Design review of the part shown in the three views and the two pictorial views. Dimensions are in mm from the part's minimum x, y and z. A direction names the side the tool comes from. Coordinates: 2 decimals unless noted, no trailing zeros. Order: outer loops, then holes, each group sorted by start corner. A loop starts at its lowest first (then second) coordinate and runs counter-clockwise, first axis right, second up. Notation, with made-up numbers: (-38, 63.5) -> (-15, 63.5) arc R16 ccw to (-15, 75.5) -> close; hole circle Ø3 at (48, 42). An arc over 180 degrees is marked (long way). Answer as a JSON object with one key per item and string values. Group by question number.
1) Draft analysis for pull direction X (two halves, no side actions). For the marked faces 1, 2 and 3, state which applies: +X half, -X half, draft (parallel to the pull), parting line (faces both ways), or undercut.
2) Add section C-C, the plane y = 29. Write out the cut boundary in (x, z), then the cut area to 3 significant figures.
3) Machinability: for the marked faces 4, 5 and 6, which of the approach directions +Z, -Z, +X, -X, +Y, -Y give a long, thin tool a straight path to every point of the face, cutting with its end or side? Answer none if there is none.
4) Add section B-B, the plane x = 58. Write out the cut boundary in (y, z).
5) Add section A-A, the plane z = 11. Write out the cut boundary in (x, y).
6) Add section D-D, the plane z = 1.5. Write out the cut boundary in (x, y), then the cut area to 3 significant figures.
7) For pin 1 (7 mm diameter, centred on x = 8, z = 7.7, fed in from +Y); pin 2 (4.5 mm diameter, centred on x = 53.5, z = 10, fed in from +Y); pin 3 (1 mm diameter, centred on y = 33.5, z = 13, fed in from +X); pin 4 (4 mm diameter, centred on x = 21.5, z = 6.5, fed in from +Y), all flat-tipped, find the tip position at first contact; note any pin that passes through.
8) Wall thickness on L1, parallel to Z at x = 58, y = 12; L2, parallel to Y at x = 33, z = 4.5; L3, parallel to X at y = 15.5, z = 11 (1 decimal): over which ranges is each line inside the solid? List them lowest first.
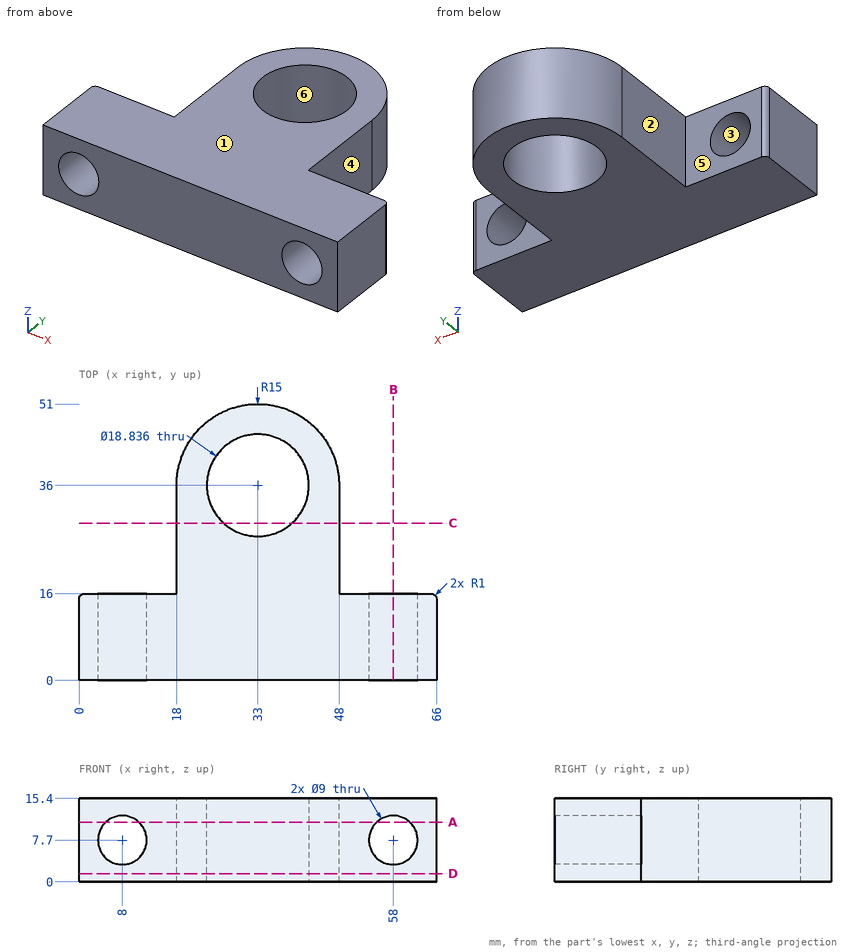
Output values:
{
 "1": {"face 1": "draft", "face 2": "-X half", "face 3": "undercut"},
 "2": {"outline": "(18, 0) -> (26.7, 0) -> (26.7, 15.4) -> (18, 15.4) -> close; (39.3, 0) -> (48, 0) -> (48, 15.4) -> (39.3, 15.4) -> close", "area": "268 mm²"},
 "3": {"face 4": "+Z, -Z, +X, +Y", "face 5": "+Z, -Z, -X, +Y", "face 6": "+Z, -Z"},
 "4": {"outline": "(0, 0) -> (16, 0) -> (16, 3.2) -> (0, 3.2) -> close; (0, 12.2) -> (16, 12.2) -> (16, 15.4) -> (0, 15.4) -> close"},
 "5": {"outline": "(0, 0) -> (4.94, 0) -> (4.94, 16) -> (1, 16) arc R1 ccw to (0, 15) -> close; (11.06, 0) -> (54.94, 0) -> (54.94, 16) -> (48, 16) -> (48, 36) arc R15 ccw to (18, 36) -> (18, 16) -> (11.06, 16) -> close; (61.06, 0) -> (66, 0) -> (66, 15) arc R1 ccw to (65, 16) -> (61.06, 16) -> close; hole circle Ø18.84 at (33, 36)"},
 "6": {"outline": "(0, 0) -> (66, 0) -> (66, 15) arc R1 ccw to (65, 16) -> (48, 16) -> (48, 36) arc R15 ccw to (18, 36) -> (18, 16) -> (1, 16) arc R1 ccw to (0, 15) -> close; hole circle Ø18.84 at (33, 36)", "area": "1,730 mm²"},
 "7": {"pin 1": "passes through", "pin 2": "stops at y = 16", "pin 3": "stops at x = 48", "pin 4": "stops at y = 47.61"},
 "8": {"L1": "z = 0 to 3.2, 12.2 to 15.4", "L2": "y = 0 to 26.58, 45.42 to 51", "L3": "x = 0.1 to 4.9, 11.1 to 54.9, 61.1 to 65.9"}
}
